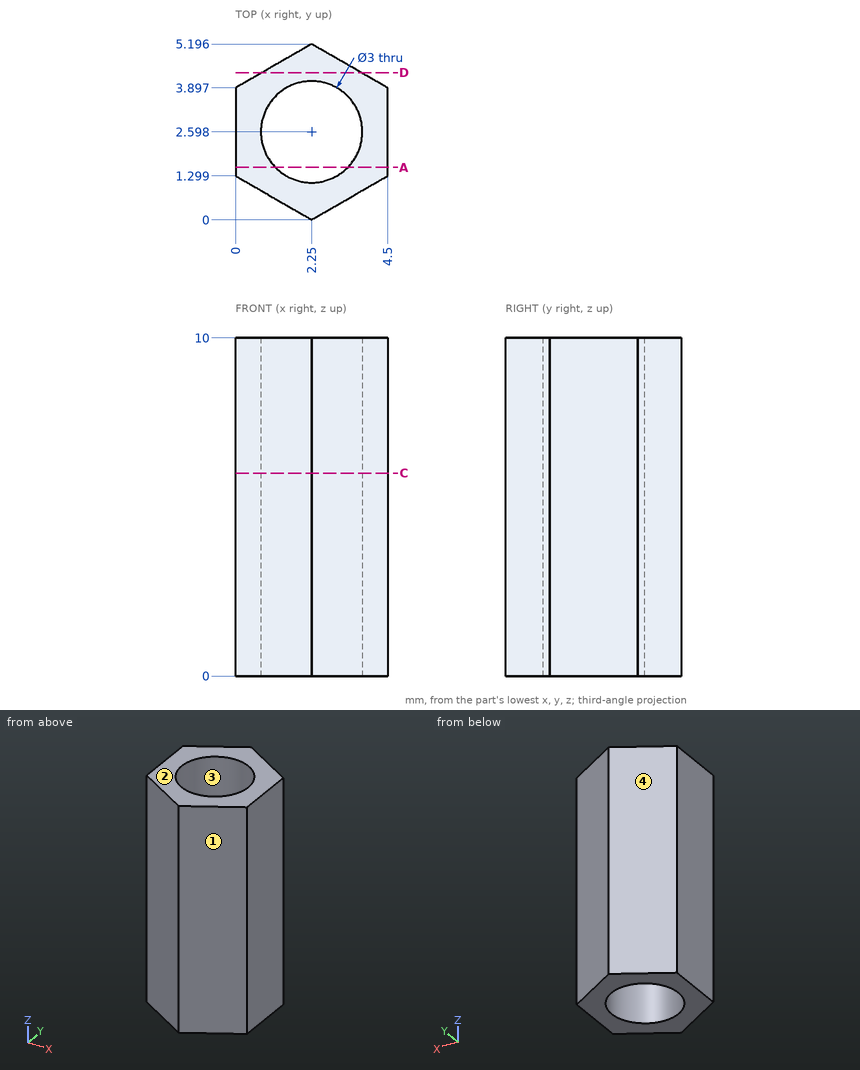
For this review, use the dimensioned drawing (mm, ordinates from the lowest corner) and the shaded views. Round coordinates to 2 decimals unless told otherwise and drop trailing zeros. Write each loop counter-clockwise with the first axis right and the second up, starting at its lowest first coordinate (ties: lowest second). Pieces come first, ordered by that corner, then holes. Notation, with made-up numbers: (-33.75, 47) -> (-9.75, 47) arc R23 ccw to (-9.75, 60) -> close; hole circle Ø10 at (-19, 22.25). An arc over 180 degrees is marked (long way). Answer in a Markdown table with one row per item.
Q1. Draft analysis for pull direction Y (two halves, no side actions). For the marked faces 1, 2, 3 and 4, state which applies: +Y half, -Y half, draft (parallel to the pull), parting line (faces both ways), or undercut.
The answers:
| item | result |
|---|---|
| face 1 | -Y half |
| face 2 | draft |
| face 3 | undercut |
| face 4 | +Y half |
Q2. Take a section at D-D, the plane y = 4.35. State the section outline as (x, z) points.
The answers:
| item | result |
|---|---|
| outline | (0.78, 0) -> (3.72, 0) -> (3.72, 10) -> (0.78, 10) -> close |
Q3. Take a section at A-A, the plane y = 1.55. State the section outline as (x, z) points.
The answers:
| item | result |
|---|---|
| outline | (0, 0) -> (1.18, 0) -> (1.18, 10) -> (0, 10) -> close; (3.32, 0) -> (4.5, 0) -> (4.5, 10) -> (3.32, 10) -> close |
Q4. To check wall thickness, follow L1, parallel to X at y = 3.75, z = 8.75; L2, parallel to X at y = 2, z = 6.75; L3, parallel to Y at x = 0.2, z = 2.5. State the ranges of each line that lie inside material, in increasing order. Write a range as [from, to].
The answers:
| item | result |
|---|---|
| L1 | [0, 1.29], [3.21, 4.5] |
| L2 | [0, 0.87], [3.63, 4.5] |
| L3 | [1.18, 4.01] |
Q5. Take a section at C-C, the plane z = 6. State the section outline as (x, y) points.
The answers:
| item | result |
|---|---|
| outline | (0, 1.3) -> (2.25, 0) -> (4.5, 1.3) -> (4.5, 3.9) -> (2.25, 5.2) -> (0, 3.9) -> close; hole circle Ø3 at (2.25, 2.6) |
